Autodesk Inventor part; units mm, degrees
ref_plane "YZ Plane" through (0, 0, 0) normal (1, 0, 0) x (0, 1, 0)
ref_plane "XZ Plane" through (0, 0, 0) normal (0, 1, 0) x (-1, 0, 0)
ref_plane "XY Plane" through (0, 0, 0) normal (0, 0, 1) x (1, 0, 0)
sketch "Sketch1" plane through (0, 0, 0) normal (0, 1, 0) x (-1, 0, 0)
  line L0 (0, 0) -> (70, 0)
  line L1 (70, 0) -> (70, -70)
  line L2 (70, -70) -> (0, -70)
  line L3 (0, -70) -> (0, 0)
  circle A0 centre (5, -5) radius 3.25
  circle A1 centre (5, -65) radius 3.25
  circle A2 centre (65, -5) radius 3.25
  circle A3 centre (65, -65) radius 3.25
  dimension "d0" = 70
  dimension "d1" = 6.5
  dimension "d4" = 60
  dimension "d7" = 60
  dimension "d10" = 5
  dimension "d11" = 5
extrude "Extrusion1" add sketch "Sketch1" along normal blind 3
fillet "Fillet1" radius 2 4 edges at (-70, 1.5, 0) (-70, 1.5, -70) (0, 1.5, -70) (0, 1.5, 0)
sketch "Sketch2" plane through (0, 3, 0) normal (0, 1, 0) x (1, 0, 0)
  line L0 (-70, 68) -> (-70, 2) construction
  line L1 (-70, 35) -> (0, 35) construction
  line L2 (0, 2) -> (0, 68) construction
  line L3 (-68, 0) -> (-2, 0) construction
  line L4 (-35, 0) -> (-35, 70) construction
  line L5 (-2, 70) -> (-68, 70) construction
  arc A0 (-35, 43.25) -> (-35, 26.75) centre (-35, 35) ccw
  arc A1 (-35, 46.25) -> (-35, 23.75) centre (-35, 35) ccw
  line L6 (-35, 23.75) -> (-35, 26.75)
  line L7 (-35, 43.25) -> (-35, 46.25)
  point P0 (0, 0)
  dimension "d17" = 8.25
  dimension "d19" = 3
revolve "Revolution1" add sketch "Sketch2" angle 180 about axis through (-35, 3, 0) along (0, 0, 1)
sketch "Sketch3" plane through (0, 3, 0) normal (0, 1, 0) x (1, 0, 0)
  circle A0 centre (-35, 35) radius 8.25
  circle A1 centre (-35, 35) radius 7.6852
  line L0 (-35, 43.25) -> (-35, 26.75)
  point P0 (0, 0)
  dimension "d40" = 16.5
revolve "Revolution2" cut sketch "Sketch3" angle 180 about axis through (-35, 3, -43.25) along (0, 0, 1) picked at (-42.6965, 37.215) picked at (-37.7213, 33.6192) contours L0 A1 A0 | L0 A1
sketch "Sketch4" plane through (0, 3, 0) normal (0, 1, 0) x (1, 0, 0)
  circle A0 centre (-35, 35) radius 7.6852
  point P0 (0, 0)
hole "Hole1" at (-35, 3, -35) direction (0, -1, 0) diameter 3 end through all
sketch "Sketch5" plane through (0, 0, 0) normal (0, -1, 0) x (1, 0, 0)
  circle A0 centre (-5, -5) radius 3.25
  circle A1 centre (-5, -5) radius 4.775
  circle A2 centre (-5, -5) radius 3.25
  line L0 (-68, 0) -> (-2, 0)
  line L1 (0, -2) -> (0, -68)
  circle A3 centre (-65, -5) radius 4.775
  circle A4 centre (-65, -5) radius 3.25
  circle A5 centre (-5, -65) radius 4.775
  circle A6 centre (-5, -65) radius 3.25
  circle A7 centre (-65, -65) radius 4.775
  circle A8 centre (-65, -65) radius 3.25
  point P0 (0, 0)
  dimension "d29" = 9.55
  dimension "d32" = 60
  dimension "d35" = 60
extrude "Extrusion2" add sketch "Sketch5" along normal blind 8
equation "\"d0\" = cradle_width"
equation "\"d1\" = rod_diameter + rod_free_tolerance"
equation "\"d4\" = rod_dist"
equation "\"d7\" = rod_dist"
equation "\"d10\" = 0.5 * cradle_width - 0.5 * rod_dist"
equation "\"d11\" = 0.5 * cradle_width - 0.5 * rod_dist"
equation "\"d12\" = cradle_holder_thickness"
equation "\"d17\" = 0.5 * tube_diameter"
equation "\"d19\" = cradle_holder_thickness"
equation "\"d40\" = tube_diameter"
equation "\"d22\" = needle_hole_diameter"
equation "\"d29\" = post_diameter - post_wall_diameter"
equation "\"d32\" = rod_dist"
equation "\"d35\" = rod_dist"
equation "\"d38\" = cradle_holder_peg_depth"
equation "\"cradle_width\" = 70"
equation "\"cradle_holder_peg_depth\" = 8"
equation "\"tube_diameter\" = 16.5"
equation "\"rod_dist\" = 60"
equation "\"rod_diameter\" = 6"
equation "\"rod_free_tolerance\" = 0.5"
equation "\"cradle_holder_thickness\" = 3"
equation "\"needle_hole_diameter\" = 3"
equation "\"post_diameter\" = 10.2"
equation "\"post_wall_diameter\" = 0.65"
properties part number "cradle_holder"
For this review, take the finished solid that the model builds, in its own axes (mm). A direction names the side the tool comes from. Give positions to 0.01 mm unless a question says otherwise; leave off trailing zeros. Write each loop counter-clockwise with the first axis right and the second up, starting at its lowest first coordinate (ties: lowest second). Pieces come first, ordered by that corner, then holes. Notation, with made-up numbers: M -13,37 L -5,37 A36 cw -5,75 Z; hole C -20.5,28 d2. An arc over 180 degrees is marked long. Answer as a JSON object with one key per item and string values. Group by question number.
Item 1: For pin 1 Ø5 at (x, z) = (-65, -65) entering from +Y; pin 2 Ø7.5 at (x, z) = (-5, -65) entering from -Y; pin 3 Ø3 at (x, y) = (-44.5, -3) entering from +Z; pin 4 Ø3.5 at (x, z) = (-35, -35) entering from +Y, all flat-tipped, find the tip position at first contact; note any pin that passes through.
Item 2: Draft analysis for pull direction X (two halves, no side actions). For faces 1 (the cylindrical face through (-0.57, 1.52, -69.4)), 2 (the flat face through (-35, 1, 0)), 3 (the cylindrical face through (-6.04, -3.94, -0.34)), state which applies: +X half, -X half, draft (parallel to the pull), parting line (faces both ways), or undercut.
Item 3: Consider section D-D on z = -5. Write out the cut boundary in (x, y) (3 decimals), plus the area to 3 significant figures.
Item 4: For probe 1 along Z at (x, y) = (-65, 1.5); probe 2 along X at (y, z) = (2, -6.5), list the stretches that pass through material, from the lowest coordinate up. Write a range as [from, to].
Item 5: Tool access review of faces 4 (the cylindrical face through (-69.43, 1.52, -0.6)), 5 (the cylindrical face through (-6.04, -3.94, -60.34)): name each direction out of +Z, -Z, +X, -X, +Y, -Y from which nothing blocks a thin tool from reaching the whole face with its end or side.
Item 6: Consider section A-A on z = -35. Write out the cut boundary in (x, y), plus the area to 3 significant figures.
Item 7: Consider section B-B on y = -6. Count the separate pieces of the cut face and the enclosed holes in it, plus the area to 3 significant figures.
Item 8: Consider section C-C on x = -35. Write out the cut boundary in (y, z).
Check result:
{
 "1": {"pin 1": "passes through", "pin 2": "stops at y = -8", "pin 3": "stops at z = -29.36", "pin 4": "stops at y = -5.06"},
 "2": {"face 1": "+X half", "face 2": "draft", "face 3": "undercut"},
 "3": {"outline": "M -70,0 L -69.775,0 L -69.775,-8 L -68.25,-8 L -68.25,3 L -70,3 Z; M -61.75,-8 L -60.225,-8 L -60.225,0 L -9.775,0 L -9.775,-8 L -8.25,-8 L -8.25,3 L -61.75,3 Z; M -1.75,-8 L -0.225,-8 L -0.225,0 L 0,0 L 0,3 L -1.75,3 Z", "area": "220 mm^2"},
 "4": {"probe 1": "z = [-70, -68.25], [-61.75, -8.25], [-1.75, 0]", "probe 2": "x = [-70, -67.88], [-62.12, -7.88], [-2.12, 0]"},
 "5": {"face 4": "+Z, -X, +Y, -Y", "face 5": "-Y"},
 "6": {"outline": "M -70,0 L -45.84,0 A11.25 ccw -36.5,-8.15 L -36.5,-5.11 A8.25 cw -43.25,3 L -70,3 Z; M -33.5,-8.15 A11.25 ccw -24.16,0 L 0,0 L 0,3 L -26.75,3 A8.25 cw -33.5,-5.11 Z", "area": "226 mm^2"},
 "7": {"separate pieces": "5", "enclosed holes": "5", "area": "290 mm^2"},
 "8": {"outline": "M -8.15,-36.5 A11.25 ccw 0,-45.84 L 0,-70 L 3,-70 L 3,-43.25 A8.25 cw -5.11,-36.5 Z; M -8.15,-33.5 L -5.11,-33.5 A8.25 cw 3,-26.75 L 3,0 L 0,0 L 0,-24.16 A11.25 ccw Z"}
}
